Verification items for the finished model (mm, model axes). A direction names the side the tool comes from. Coordinates: 2 decimals unless noted, no trailing zeros. Loops run counter-clockwise (first coordinate to the right, second up) from the corner with the lowest first, then second, coordinate; pieces in that order, holes last.
Q1. Go/stop test with flat-tipped pins: P1, Ø1, axis at x = -2, z = 39.5, coming from the -Y side; P2, Ø2, axis at x = -2, z = 13, coming from the -Y side. Record where each tip stops, or that it passes through.
Q2. Sectioned sample at B-B (z = 59.5). Enter the section's corners in (x, y).
Q3. Material ranges on probe 1 along Z at (x, y) = (1.75, 0.5); probe 2 along Z at (x, y) = (0.25, 5.25); probe 3 along Y at (x, z) = (2.5, 38), recorded low to high.
Q4. Sectioned sample at A-A (z = 33.5). Enter the section's corners in (x, y).
Q5. Access from +Z, -Z, +X, -X, +Y, -Y to the whole of each face (thin tool, end or side, straight path). Record for faces 1 (the face through (2, 0, 63.373)), 2 (the face through (-2, 0, 63.5)), 3 (the face through (0, 5.08, 54)).
```python
from build123d import *

# Parameters (mm, degrees)
SKETCH1_R                     = 6.34365
MAIN_SHAFTBOSS_EXTRUDE1_DEPTH = 63.5
SKETCH2_W                     = 9.398
SKETCH2_H                     = 3.175
SHAFT_FLATCUT_EXTRUDE1_DEPTH  = 19.05
CHAMFER1_SIZE                 = 0.508
SKETCH3_W                     = 7.358407373
SKETCH3_H                     = 13.78482206
FACETARGETCUT_EXTRUDE2_DEPTH  = 0.127


with BuildPart() as part:
    # Sketch1 → Main ShaftBoss-Extrude1 (new body)
    with BuildSketch(Plane.XY):
        Circle(SKETCH1_R)
    extrude(amount=MAIN_SHAFTBOSS_EXTRUDE1_DEPTH)

    # Sketch2 → Shaft FlatCut-Extrude1 (cut)
    with BuildSketch(Plane.XY.offset(63.5)):
        with Locations((0, 6.6675)):
            Rectangle(SKETCH2_W, SKETCH2_H)
    extrude(amount=-SHAFT_FLATCUT_EXTRUDE1_DEPTH, mode=Mode.SUBTRACT)

    # Chamfer1
    chamfer1_edges = [part.edges().sort_by_distance(p)[0] for p in [
        (-6.34365, 0, 0),
        (-2.840755677, -5.672036892, 63.5),
    ]]
    chamfer(chamfer1_edges, length=CHAMFER1_SIZE)

    # Sketch3 → FaceTargetCut-Extrude2 (cut)
    with BuildSketch(Plane.XY.offset(63.5)):
        with Locations((3.679203687, -0.119208367)):
            Rectangle(SKETCH3_W, SKETCH3_H)
    extrude(amount=-FACETARGETCUT_EXTRUDE2_DEPTH, mode=Mode.SUBTRACT)


solid = part.part
```
Geometry check:
1. P1: stops at y = -6.16
1. P2: stops at y = -6.26
2. outline: (-3.8, 5.08) arc R6.34 ccw (long way) to (3.8, 5.08) - close
3. probe 1: z = 0 to 63.37
3. probe 2: z = 0 to 44.45
3. probe 3: y = -5.83 to 5.83
4. outline: circle Ø12.69 at (0, 0)
5. face 1: +Z, +X, +Y, -Y
5. face 2: +Z, +X, -X, +Y, -Y
5. face 3: +Z, +X, -X, +Y
